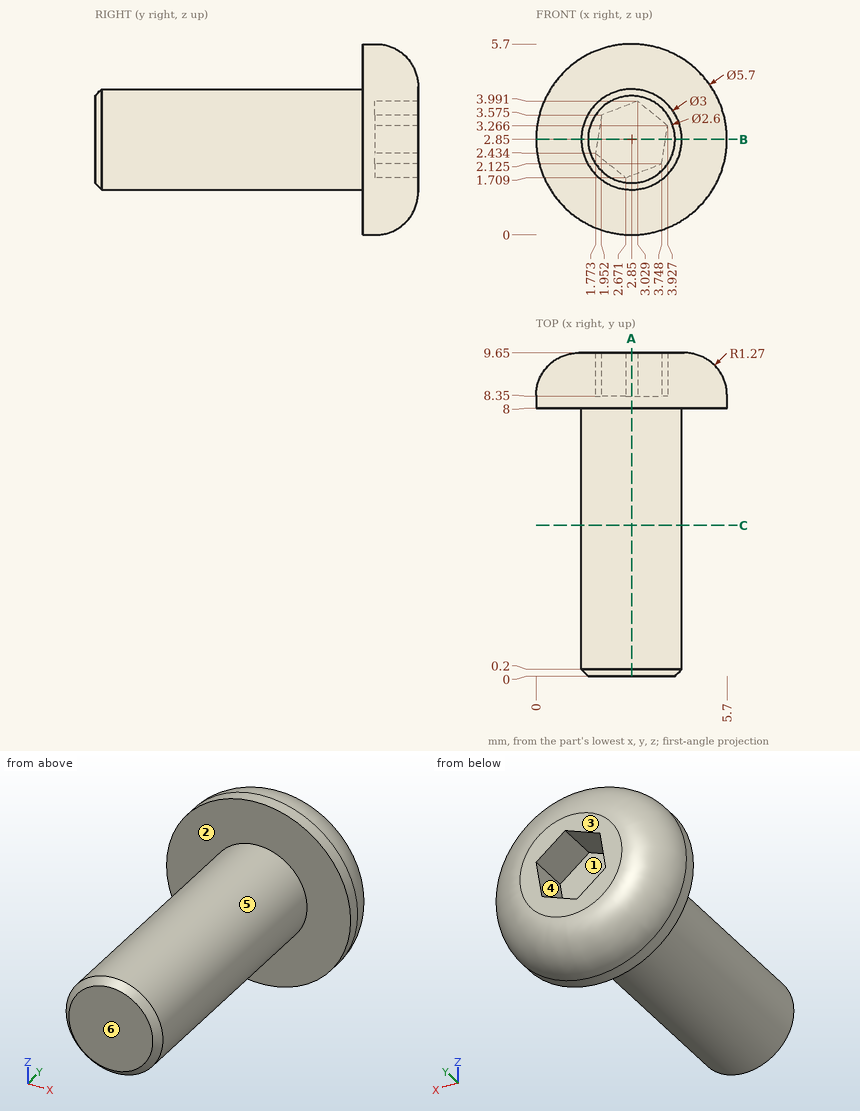
Here's the drawing with two shaded views (mm, measured from the low corner). I have some questions. A direction names the side the tool comes from. Coordinates: 2 decimals unless noted, no trailing zeros. Write each loop counter-clockwise with the first axis right and the second up, starting at its lowest first coordinate (ties: lowest second). Pieces come first, ordered by that corner, then holes.
Item 1: I want a section at A-A on x = 2.85. Write out the boundary of the cut face in (y, z), and give its area (3 significant figures).
Item 2: I want a section at B-B on z = 2.85. Write out the boundary of the cut face in (x, y).
Item 3: If I drill on line 1 (Y direction, x = 2.15, z = 2.3); line 2 (Z direction, x = 2.1, y = 0.5); line 3 (X direction, y = 8.5, z = 2.6), over which ranges is the centre line in solid material (lowest first)?
Item 4: Will these pins go through, and if not, where does the flat tip stop? pin 1 (1.5 mm diameter, centred on y = 5.5, z = 4, fed in from -X) (1 decimal); pin 2 (0.6 mm diameter, centred on x = 3, z = 2.5, fed in from +Y); pin 3 (1 mm diameter, centred on x = 4, y = 3.5, fed in from -Z).
Item 5: If we mould it in two halves opening along X, with no side actions, what happens to the marked faces 4, 5 and 6? For each: +X half, -X half, draft (parallel to the pull), parting line (faces both ways), or undercut.
Item 6: I want a section at C-C on y = 4.5. Write out the boundary of the cut face in (x, z).
Item 7: On a 3-axis mill with a long thin cutter (end or side, diameter ignored), from which of +Z, -Z, +X, -X, +Y, -Y can I reach the whole of each face in a straight line? I mean the marked faces 1, 2 and 3. Say none if no direction works.
Findings below:
1. outline: (0, 1.55) - (0.2, 1.35) - (8, 1.35) - (8, 0) - (8.38, 0) arc R1.27 ccw to (9.65, 1.27) - (9.65, 1.78) - (8.35, 1.78) - (8.35, 3.92) - (9.65, 3.92) - (9.65, 4.43) arc R1.27 ccw to (8.38, 5.7) - (8, 5.7) - (8, 4.35) - (0.2, 4.35) - (0, 4.15) - close
1. area: 29.9 mm2
2. outline: (0, 8) - (1.35, 8) - (1.35, 0.2) - (1.55, 0) - (4.15, 0) - (4.35, 0.2) - (4.35, 8) - (5.7, 8) - (5.7, 8.38) arc R1.27 ccw to (4.43, 9.65) - (3.86, 9.65) - (3.86, 8.35) - (1.84, 8.35) - (1.84, 9.65) - (1.27, 9.65) arc R1.27 ccw to (0, 8.38) - close
3. line 1: y = 0 to 8.35
3. line 2: z = 1.55 to 4.15
3. line 3: x = 0.02 to 1.8, 3.82 to 5.68
4. pin 1: stops at x = 1.4
4. pin 2: stops at y = 8.35
4. pin 3: stops at z = 1.5
5. face 4: undercut
5. face 5: parting line
5. face 6: draft
6. outline: circle Ø3 at (2.85, 2.85)
7. face 1: +Y
7. face 2: -Y
7. face 3: +Z, -Z, +X, -X, +Y
